Autodesk Inventor part; units mm, degrees
ref_plane "YZ Plane" through (0, 0, 0) normal (1, 0, 0) x (0, 1, 0)
ref_plane "XZ Plane" through (0, 0, 0) normal (0, 1, 0) x (-1, 0, 0)
ref_plane "XY Plane" through (0, 0, 0) normal (0, 0, 1) x (1, 0, 0)
sketch "Sketch1" plane through (0, 0, 0) normal (0, 0, 1) x (1, 0, 0)
  circle A0 centre (-48, 0) radius 1
  circle A1 centre (48, 0) radius 1
  line L0 (-48, 0) -> (0, 0) construction
  line L1 (0, 0) -> (48, 0) construction
  line L2 (-48, 3) -> (48, 3)
  line L3 (-48, -3) -> (48, -3)
  line L4 (0, 3) -> (0, -3) construction
  arc A2 (-48, 3) -> (-48, -3) centre (-48, 0) ccw
  arc A3 (48, -3) -> (48, 3) centre (48, 0) ccw
  circle A4 centre (-38, 0) radius 1
  circle A5 centre (-38, -6) radius 3
  line L5 (-41, -6) -> (-41, -3)
  line L6 (-35, -6) -> (-35, -3)
  circle A6 centre (-38, -6) radius 1
  point P0 (-48, -1)
  dimension "d0" = 2
  dimension "d1" = 2
  dimension "d2" = 48
  dimension "d5" = 10
extrude "Extrusion1" add sketch "Sketch1" along normal blind 2
properties part number "Wing"
The listing builds one solid part. Answer for the finished solid, in the listing's coordinates (mm). A direction names the side the tool comes from. Give positions to 0.01 mm unless a question says otherwise; leave off trailing zeros. Order: outer loops, then holes, each group sorted by start corner. A loop starts at its lowest first (then second) coordinate and runs counter-clockwise, first axis right, second up. Notation, with made-up numbers: (68.5, 25.5) - (111.5, 25.5) arc R17 cw to (111.5, 56.5) - close; hole circle Ø4 at (65.25, 33). An arc over 180 degrees is marked (long way). One line per item, written item: value. Start each with the question number.
1) Find the intervals of material crossed by L1, parallel to Y at x = -38, z = 1.5; L2, parallel to Y at x = -48, z = 1.2; L3, parallel to Y at x = -23, z = 0.85, in increasing order.
2) The mould has two halves that part along X. Classify faces 4 (the face through (-37, -6, 1)), 5 (the face through (-1, 0, 2)), 6 (the face through (-41, -5, 1)): released by +X, released by -X, zero draft, split by the parting line, or undercut.
3) Given pin 1 Ø0.6 at (x, z) = (8, 1.5) entering from -Y; pin 2 Ø0.6 at (y, z) = (-4.5, 0.5) entering from +X; pin 3 Ø1.6 at (x, y) = (-48, 0) entering from -Z; pin 4 Ø1 at (y, z) = (-4.5, 0.5) entering from -X, each flat-ended and moving along its own axis, determine where each tip first touches the part or whether it passes through.
4) A tool of negligible diameter and unlimited length cuts with its end or side. For faces 1 (the face through (-45, -3, 1)), 2 (the face through (-35, -5, 1)), 3 (the face through (-1, 3, 1)), from which of +Z, -Z, +X, -X, +Y, -Y can it reach the whole face along a straight path? Write none if from no direction.
5) A cutting plane is placed at A-A on y = 0. Give the vertices of the cut face in (x, z), then the cut area to 3 significant figures.
6) A cutting plane is placed at B-B on x = -38. Give the vertices of the cut face in (y, z), then the cut area to 3 significant figures.
7) A cutting plane is placed at C-C on x = -4. Give the vertices of the cut face in (y, z), then the cut area to 3 significant figures.
Answer sheet:
1. L1: y = -9 to -7, -5 to -1, 1 to 3
1. L2: y = -3 to -1, 1 to 3
1. L3: y = -3 to 3
2. face 4: undercut
2. face 5: zero draft
2. face 6: released by -X
3. pin 1: stops at y = -3
3. pin 2: stops at x = -35
3. pin 3: passes through
3. pin 4: stops at x = -41
4. face 1: +Z, -Z, -X, -Y
4. face 2: +Z, -Z, +X, -Y
4. face 3: +Z, -Z, +X, -X, +Y
5. outline: (-51, 0) - (-49, 0) - (-49, 2) - (-51, 2) - close; (-47, 0) - (-39, 0) - (-39, 2) - (-47, 2) - close; (-37, 0) - (47, 0) - (47, 2) - (-37, 2) - close; (49, 0) - (51, 0) - (51, 2) - (49, 2) - close
5. area: 192 mm2
6. outline: (-9, 0) - (-7, 0) - (-7, 2) - (-9, 2) - close; (-5, 0) - (-1, 0) - (-1, 2) - (-5, 2) - close; (1, 0) - (3, 0) - (3, 2) - (1, 2) - close
6. area: 16.0 mm2
7. outline: (-3, 0) - (3, 0) - (3, 2) - (-3, 2) - close
7. area: 12.0 mm2
